For this review, take the finished solid that the model builds, in its own axes (mm). A direction names the side the tool comes from. Coordinates: 2 decimals unless noted, no trailing zeros. Write each loop counter-clockwise with the first axis right and the second up, starting at its lowest first coordinate (ties: lowest second). Pieces come first, ordered by that corner, then holes.
1) We need section C-C on x = 6.5. Write out the cut boundary in (y, z), then the cut area to 3 significant figures.
2) Insertion check: P1, Ø0.6, axis at x = 1.5, z = 9, coming from the -Y side; P2, Ø1.6, axis at x = -19, y = -26.5, coming from the -Z side; P3, Ø1.6, axis at y = -27, z = -5, coming from the -X side. Each pin has a flat end and moves straight along its axis. Give the tip position at first contact, or say it passes through.
3) For faces 1 (the face through (32, -13, -7)), 2 (the face through (-15.5, 18, 9)), 3 (the face through (-9.5, -26, -6)), 4 (the face through (-31.93, 0.36, 9.4)), 5 (the face through (30.5, 0, -1)), list the 3-axis set-ups (+Z, -Z, +X, -X, +Y, -Y) from which the entire face can be reached by the end or side of a thin tool; tool diameter is ignored.
4) Mouldability with a two-part tool opening along Y and no side actions: class faces 6 (the face through (-31.93, -26.9, -0.87)), 7 (the face through (-23, 23.5, 9)), 8 (the face through (0.43, 26.93, 9.4)) as pulls with the +Y half, pulls with the -Y half, needs draft (parallel to the pull), parting line crosses it, or undercut.
5) To check wall thickness, follow line 1 along Y through (x, z) = (11.5, 6.75); line 2 along X through (y, z) = (7, 1); line 3 along Z through (x, y) = (-23, -17). State the ranges of each line that lie inside material, in increasing order.
6) We need section D-D on y = -3. Write out the cut boundary in (x, z).
from build123d import *

# Parameters (mm, degrees)
F0_W     = 65
F0_H     = 55
F1_DEPTH = 10
F2_T     = -2
F3_W     = 17
F3_H     = 17
F3_W_2   = 15
F3_H_2   = 9
F4_DEPTH = 27.5
F6_DEPTH = 25.4
F7_W     = 15
F7_H     = 10
F7_W_2   = 18
F7_H_2   = 4
F8_DEPTH = 12.7
F9_R     = 1.99999


# Not quite as in the source:
# - a fillet or chamfer is up to 0.001 mm smaller than in the source, because OpenCascade refuses the exact size


with BuildPart() as f1:
    # F0 (on Top) → F1 (new body, symmetric)
    with BuildSketch(Plane.XY):
        Rectangle(F0_W, F0_H)
    extrude(amount=F1_DEPTH, both=True)

    # F2
    f2_openings = [f1.faces().sort_by_distance(p)[0] for p in [
        (0, 0, -10),
    ]]
    offset(amount=F2_T, openings=f2_openings)

    # F3 (on Front) → F4 (cut, through all)
    with BuildSketch(Plane.XZ):
        with Locations((-22, -1.5)):
            Rectangle(F3_W, F3_H)
        with Locations((-2, -5.5)):
            Rectangle(F3_W_2, F3_H_2)
    extrude(amount=F4_DEPTH, mode=Mode.SUBTRACT)

    # F5 (on face) → F6 (cut)
    with BuildSketch(Plane.YZ.offset(32.5)):
        with BuildLine():
            Line((-14.5, -10), (-13, -10))
            ThreePointArc((-13, -10), (-14.0606601718, -9.5606601718), (-14.5, -8.5))
            Line((-14.5, -8.5), (-14.5, -10))
        make_face()
        with BuildLine():
            ThreePointArc((-13, -10), (-11.9393398282, -9.5606601718), (-11.5, -8.5))
            ThreePointArc((-11.5, -8.5), (-11.5000361058, -8.4895924938), (-11.5001444216, -8.4791854886))
            ThreePointArc((-11.5001444216, -8.4791854886), (-13.0104075062, -7.0000361058), (-14.5, -8.5))
            ThreePointArc((-14.5, -8.5), (-14.0606601718, -9.5606601718), (-13, -10))
        make_face()
        with BuildLine():
            ThreePointArc((-11.5001444216, -8.4791854886), (-11.5000361058, -8.4895924938), (-11.5, -8.5))
            ThreePointArc((-11.5, -8.5), (-11.9393398282, -9.5606601718), (-13, -10))
            Line((-13, -10), (-11.4790390489, -10))
            Line((-11.4790390489, -10), (-11.5001444216, -8.4791854886))
        make_face()
        with BuildLine():
            ThreePointArc((-6.5, -8.5), (-8, -7), (-9.5, -8.5))
            ThreePointArc((-9.5, -8.5), (-9.0606601747, -9.5606601688), (-8.0000000084, -10))
            ThreePointArc((-8.0000000084, -10), (-6.9393398312, -9.5606601747), (-6.5, -8.5))
        make_face()
        with BuildLine():
            Line((-9.5, -8.5), (-9.5, -10))
            Line((-9.5, -10), (-8.0000000084, -10))
            ThreePointArc((-8.0000000084, -10), (-9.0606601747, -9.5606601688), (-9.5, -8.5))
        make_face()
        with BuildLine():
            ThreePointArc((-6.5, -8.5), (-6.9393398312, -9.5606601747), (-8.0000000084, -10))
            Line((-8.0000000084, -10), (-6.5, -10))
            Line((-6.5, -10), (-6.5, -8.5))
        make_face()
        with BuildLine():
            ThreePointArc((-1.5, -8.5), (-3, -7), (-4.5, -8.5))
            ThreePointArc((-4.5, -8.5), (-4.0606601718, -9.5606601718), (-3, -10))
            ThreePointArc((-3, -10), (-1.9393398282, -9.5606601718), (-1.5, -8.5))
        make_face()
        with BuildLine():
            Line((-4.5, -8.5), (-4.5, -10))
            Line((-4.5, -10), (-3, -10))
            ThreePointArc((-3, -10), (-4.0606601718, -9.5606601718), (-4.5, -8.5))
        make_face()
        with BuildLine():
            ThreePointArc((-1.5, -8.5), (-1.9393398282, -9.5606601718), (-3, -10))
            Line((-3, -10), (-1.5, -10))
            Line((-1.5, -10), (-1.5, -8.5))
        make_face()
    extrude(amount=-F6_DEPTH, mode=Mode.SUBTRACT)

    # F7 (on face) → F8 (cut, symmetric)
    with BuildSketch(Plane.XY.offset(10)):
        with Locations((-23, 18.5)):
            Rectangle(F7_W, F7_H)
        with Locations((-1.5, -17.5)):
            Rectangle(F7_W_2, F7_H_2)
    extrude(amount=F8_DEPTH, both=True, mode=Mode.SUBTRACT)

    # F9 (radius 2 in the source; OpenCascade refuses exactly that, so slightly less here)
    f9_edges = [f1.edges().sort_by_distance(p)[0] for p in [
        (-32.5, -27.5, 0),
        (32.5, -27.5, 0),
        (32.5, 27.5, 0),
        (-32.5, 27.5, 0),
        (0, -27.5, 10),
        (32.5, 0, 10),
        (0, 27.5, 10),
        (-32.5, 0, 10),
    ]]
    fillet(f9_edges, radius=F9_R)


solid = f1.part
Result:
1. outline: (-27.5, -10) - (-25.5, -10) - (-25.5, 8) - (-19.5, 8) - (-19.5, 10) - (-25.5, 10) arc R2 ccw to (-27.5, 8) - close; (-15.5, 8) - (25.5, 8) - (25.5, -10) - (27.5, -10) - (27.5, 8) arc R2 ccw to (25.5, 10) - (-15.5, 10) - close
1. area: 172 mm2
2. P1: stops at y = -27.37
2. P2: stops at z = 7
2. P3: stops at x = -32.37
3. face 1: -Z, +X
3. face 2: +Z, -Z
3. face 3: -Z, -Y
3. face 4: +Z, -X, +Y, -Y
3. face 5: -Z
4. face 6: pulls with the -Y half
4. face 7: undercut
4. face 8: pulls with the +Y half
5. line 1: y = -27.5 to -25.5, 25.5 to 27.5
5. line 2: x = -32.5 to -30.5, 30.5 to 32.5
5. line 3: z = 8 to 10
6. outline: (-32.5, -10) - (-30.5, -10) - (-30.5, 8) - (30.5, 8) - (30.5, -7) - (32.5, -7) - (32.5, 8) arc R2 ccw to (30.5, 10) - (-30.5, 10) arc R2 ccw to (-32.5, 8) - close
